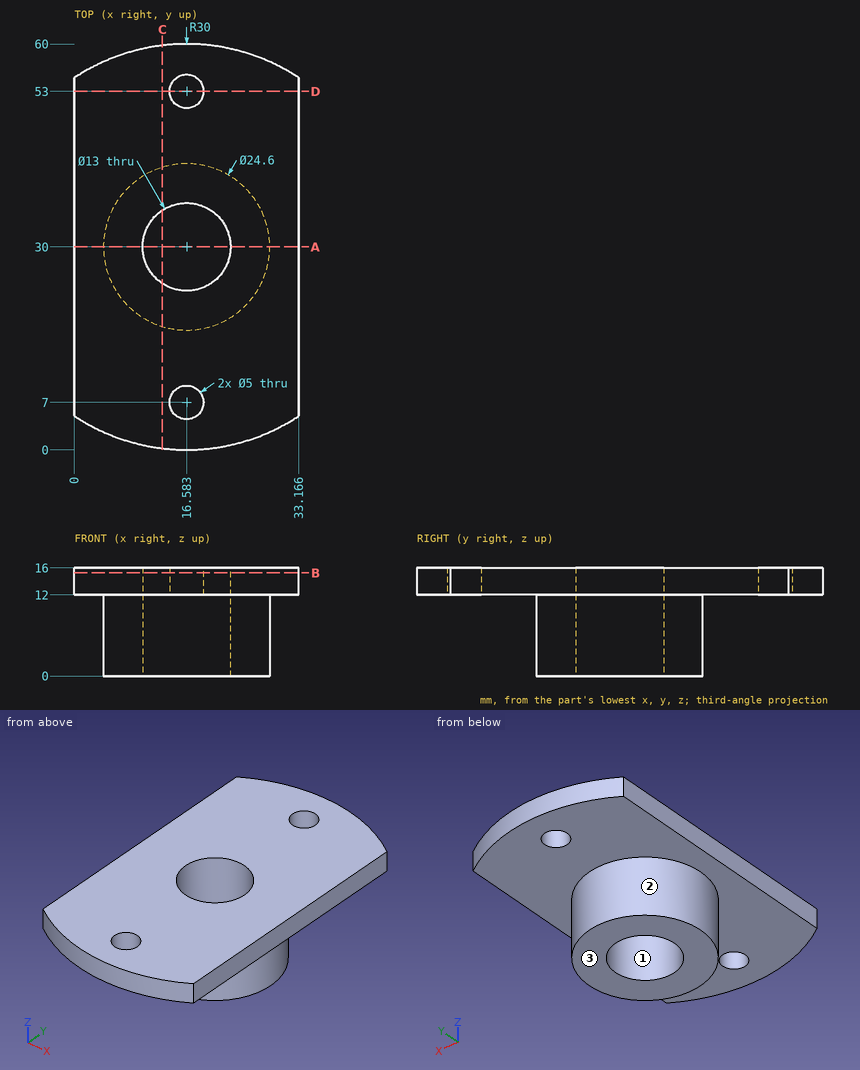
Could you check a few things on this drawing? It's one solid part, dimensions in mm from its lowest x, y, z. Coordinates: 2 decimals unless noted, no trailing zeros. Write each loop counter-clockwise with the first axis right and the second up, starting at its lowest first coordinate (ties: lowest second). Pieces come first, ordered by that corner, then holes.
1) If we section it at B-B (z = 15.25): List the corners of the cut face in (x, y) for me, plus the area to 3 significant figures.
Filled in:
outline: (0, 5) arc R30 ccw to (33.17, 5) - (33.17, 55) arc R30 ccw to (0, 55) - close; hole circle Ø13 at (16.58, 30); hole circle Ø5 at (16.58, 7); hole circle Ø5 at (16.58, 53)
area: 1,710 mm2
2) If we section it at C-C (x = 13): List the corners of the cut face in (y, z) for me (1 decimal).
Filled in:
outline: (0.2, 12) - (18.2, 12) - (18.2, 0) - (24.6, 0) - (24.6, 16) - (0.2, 16) - close; (35.4, 0) - (41.8, 0) - (41.8, 12) - (59.8, 12) - (59.8, 16) - (35.4, 16) - close
3) If we section it at D-D (y = 53): List the corners of the cut face in (x, z) for me, plus the area to 3 significant figures.
Filled in:
outline: (0, 12) - (14.08, 12) - (14.08, 16) - (0, 16) - close; (19.08, 12) - (33.17, 12) - (33.17, 16) - (19.08, 16) - close
area: 113 mm2
4) I'm going to push flat-ended pins straight in: pin 1 (6 mm diameter, centred on x = 12.5, z = 4, fed in from -Y); pin 2 (11.5 mm diameter, centred on x = 16.58, y = 30, fed in from +Z); pin 3 (2 mm diameter, centred on x = 28.5, y = 47.5, fed in from -Z); pin 4 (1.5 mm diameter, centred on x = 11.5, z = 9, fed in from -Y). Where does each tip first touch, or does it pass through?
Filled in:
pin 1: stops at y = 17.75
pin 2: passes through
pin 3: stops at z = 12
pin 4: stops at y = 18.49
5) Thinking about a two-plate mould opening in Y: for the marked faces 1, 2 and 3, which applies, +Y half, -Y half, draft (parallel to the pull), parting line (faces both ways), or undercut?
Filled in:
face 1: undercut
face 2: parting line
face 3: draft
6) If we section it at A-A (y = 30): List the corners of the cut face in (x, z) for me, plus the area to 3 significant figures.
Filled in:
outline: (0, 12) - (4.28, 12) - (4.28, 0) - (10.08, 0) - (10.08, 16) - (0, 16) - close; (23.08, 0) - (28.88, 0) - (28.88, 12) - (33.17, 12) - (33.17, 16) - (23.08, 16) - close
area: 220 mm2
7) If I drill on line 1 (Z direction, x = 8, y = 44); line 2 (X direction, y = 30, z = 11.5); line 3 (X direction, y = 7, z = 13.85), over which ranges is the centre line in solid material (lowest first)?
Filled in:
line 1: z = 12 to 16
line 2: x = 4.28 to 10.08, 23.08 to 28.88
line 3: x = 0 to 14.08, 19.08 to 33.17
